Could you check a few things on this model? Use its own coordinates, in mm. A direction names the side the tool comes from. Give positions to 0.01 mm unless a question says otherwise; leave off trailing zeros. Write each loop counter-clockwise with the first axis right and the second up, starting at its lowest first coordinate (ties: lowest second). Pieces come first, ordered by that corner, then holes. Notation, with made-up numbers: M 18,38 L 48,38 A36 ccw 48,75 Z; hole C 40.5,-12.75 d5. An arc over 180 degrees is marked long. One line per item, written item: value.
```python
from build123d import *

# Parameters (mm, degrees)
ESQUISSE1_W             = 52
ESQUISSE1_H             = 44.3
BOSS_EXTRU_1_DEPTH      = 22.3
ESQUISSE4_W             = 38.9
ESQUISSE4_H             = 16.9
ENL_V_MAT_EXTRU_2_DEPTH = 52
BOSS_EXTRU_3_DEPTH      = 44.3
ESQUISSE9_W             = 5.32335475
ESQUISSE9_H             = 32.7
BOSS_EXTRU_4_DEPTH      = 4
ESQUISSE10_W            = 32.7
ESQUISSE10_H            = 4
BOSS_EXTRU_5_DEPTH      = 14.5
ESQUISSE11_W            = 6.122616958
ESQUISSE11_H            = 32.7
BOSS_EXTRU_6_DEPTH      = 4
ESQUISSE12_W            = 32.660291113
ESQUISSE12_H            = 4
BOSS_EXTRU_7_DEPTH      = 14.5
CONG_1_R                = 10
CONG_2_R                = 10
CONG_3_R                = 10
CONG_4_R                = 10


with BuildPart() as part:
    # Esquisse1 → Boss.-Extru.1 (new body)
    with BuildSketch(Plane(origin=(0, 0, 0), x_dir=(1, 0, 0), z_dir=(0, 1, 0))):
        with Locations((-7.759163987, 0)):
            Rectangle(ESQUISSE1_W, ESQUISSE1_H)
    extrude(amount=BOSS_EXTRU_1_DEPTH)

    # Esquisse4 → Enlèv. mat.-Extru.2 (cut)
    with BuildSketch(Plane(origin=(18.240836013, 0, 0), x_dir=(0, 0, -1), z_dir=(1, 0, 0))):
        with Locations((0, 11.15)):
            Rectangle(ESQUISSE4_W, ESQUISSE4_H)
    extrude(amount=-ENL_V_MAT_EXTRU_2_DEPTH, mode=Mode.SUBTRACT)

    # Esquisse5 → Boss.-Extru.3 (add)
    with BuildSketch(Plane.XY.offset(22.15)):
        with BuildLine():
            Line((-33.759163987, 22.3), (-33.759163987, 0))
            ThreePointArc((-33.759163987, 0), (-44.909163987, 11.15), (-33.759163987, 22.3))
        make_face()
    extrude(amount=-BOSS_EXTRU_3_DEPTH)

    # Esquisse9 → Boss.-Extru.4 (add)
    with BuildSketch(Plane.XZ):
        with Locations((15.579158638, 0)):
            Rectangle(ESQUISSE9_W, ESQUISSE9_H)
    extrude(amount=BOSS_EXTRU_4_DEPTH)

    # Esquisse10 → Boss.-Extru.5 (add)
    with BuildSketch(Plane(origin=(18.240836013, 0, 0), x_dir=(0, 0, -1), z_dir=(1, 0, 0))):
        with Locations((0, -2)):
            Rectangle(ESQUISSE10_W, ESQUISSE10_H)
    extrude(amount=BOSS_EXTRU_5_DEPTH)

    # Esquisse11 → Boss.-Extru.6 (add)
    with BuildSketch(Plane(origin=(0, 22.3, 0), x_dir=(1, 0, 0), z_dir=(0, 1, 0))):
        with Locations((15.179527534, 0)):
            Rectangle(ESQUISSE11_W, ESQUISSE11_H)
    extrude(amount=BOSS_EXTRU_6_DEPTH)

    # Esquisse12 → Boss.-Extru.7 (add)
    with BuildSketch(Plane(origin=(18.240836013, 0, 0), x_dir=(0, 0, -1), z_dir=(1, 0, 0))):
        with Locations((0.019854443, 24.3)):
            Rectangle(ESQUISSE12_W, ESQUISSE12_H)
    extrude(amount=BOSS_EXTRU_7_DEPTH)

    # Congé1
    # the kernel refuses this fillet: 10 mm, written as the material it takes off along each edge
    with BuildSketch(Plane(origin=(12.917481263, -4, -36.35), x_dir=(1, 0, 0), z_dir=(0, 0, 1))) as cong_1_piece_1:
        with BuildLine():
            CenterArc((8, 10), CONG_1_R, 216.869897646, 53.130102354)
            Line((0, 4), (-0.16, 3.88))
            ThreePointArc((-0.16, 3.88), (-0.2, 2), (-0.2, 0))
            Line((-0.2, 0), (0, -0.2))
            Line((0, -0.2), (8, -0.2))
            Line((8, -0.2), (8, 0))
        make_face()
    extrude(amount=72.7, mode=Mode.SUBTRACT)

    # Congé2
    # the kernel refuses this fillet: 10 mm, written as the material it takes off along each edge
    with BuildSketch(Plane(origin=(12.118219055, 26.3, 36.35), x_dir=(1, 0, 0), z_dir=(0, 0, -1))) as cong_2_piece_1:
        with BuildLine():
            CenterArc((8, 10), CONG_2_R, 216.869897646, 53.130102354)
            Line((0, 4), (-0.16, 3.88))
            ThreePointArc((-0.16, 3.88), (-0.2, 2), (-0.2, 0))
            Line((-0.2, 0), (0, -0.2))
            Line((0, -0.2), (8, -0.2))
            Line((8, -0.2), (8, 0))
        make_face()
    extrude(amount=72.7, mode=Mode.SUBTRACT)

    # Congé3
    # the kernel refuses this fillet: 10 mm, written as the material it takes off along each edge
    with BuildSketch(Plane(origin=(32.740836013, -4, -36.35), x_dir=(-1, 0, 0), z_dir=(0, 0, 1))) as cong_3_piece_1:
        with BuildLine():
            CenterArc((8, -10), CONG_3_R, 90, 53.130102354)
            Line((0, -4), (-0.16, -3.88))
            ThreePointArc((-0.16, -3.88), (-0.2, -2), (-0.2, 0))
            Line((-0.2, 0), (0, 0.2))
            Line((0, 0.2), (8, 0.2))
            Line((8, 0.2), (8, 0))
        make_face()
    extrude(amount=72.7, mode=Mode.SUBTRACT)

    # Congé4
    # the kernel refuses this fillet: 10 mm, written as the material it takes off along each edge
    with BuildSketch(Plane(origin=(32.740836013, 26.3, -36.35), x_dir=(0, -1, 0), z_dir=(0, 0, 1))) as cong_4_piece_1:
        with BuildLine():
            CenterArc((10, -8), CONG_4_R, 126.869897646, 53.130102354)
            Line((0, -8), (-0.2, -8))
            Line((-0.2, -8), (-0.2, 0))
            Line((-0.2, 0), (0, 0.2))
            ThreePointArc((0, 0.2), (2, 0.2), (3.88, 0.16))
            Line((3.88, 0.16), (4, 0))
        make_face()
    extrude(amount=72.660291113, mode=Mode.SUBTRACT)


solid = part.part
```
1) We'd pull the mould along Z, two halves only. Please class faces 6 (the face through (23, -2, 16.35)), 7 (the face through (23, -4, 0)), 8 (the face through (-7, 2.7, 0)): pulls with the +Z half, pulls with the -Z half, needs draft (parallel to the pull), parting line crosses it, or undercut.
Outcome:
face 6: pulls with the +Z half
face 7: needs draft
face 8: undercut
2) On a 3-axis mill with a long thin cutter (end or side, diameter ignored), from which of +Z, -Z, +X, -X, +Y, -Y can I reach the whole of each face in a straight line? I mean faces 1 (the face through (23, -2, -16.35)), 2 (the face through (16.387, -2.915, -0.229)), 3 (the face through (22, 24, -16.35)), 4 (the face through (-33.759, 11, 0)), 5 (the face through (25, 22.3, 0)). Say none if no direction works.
Outcome:
face 1: -Z, +X, -X, -Y
face 2: +Z, -Z, -X, -Y
face 3: -Z, +X, -X, +Y
face 4: +X
face 5: +Z, -Z, +X
3) If we section it at C-C, the plane z = -15.5: Write out the boundary of the cut face in (x, y).
Outcome:
outline: M -33.76,0 L 12.92,0 A10 ccw 20.92,-4 L 24.74,-4 A10 ccw 32.74,0 L 18.24,0 L 18.24,2.7 L -33.76,2.7 L -33.76,19.6 L 18.24,19.6 L 18.24,22.3 L 32.74,22.3 A10 ccw 24.74,26.3 L 20.12,26.3 A10 ccw 12.12,22.3 L -33.76,22.3 A11.15 ccw Z
4) If we section it at D-D, the plane y = 11.15: Write out the boundary of the cut face in (x, z), then the cut area to 3 significant figures.
Outcome:
outline: M -44.91,-22.15 L 18.24,-22.15 L 18.24,-19.45 L -33.76,-19.45 L -33.76,19.45 L 18.24,19.45 L 18.24,22.15 L -44.91,22.15 Z
area: 775 mm^2
5) If we section it at A-A, the plane x = 23.5: Write out the boundary of the cut face in (y, z), then the cut area to 3 significant figures.
Outcome:
outline: M -4,-16.35 L 0,-16.35 L 0,16.35 L -4,16.35 Z; M 22.3,-16.35 L 26.3,-16.35 L 26.3,16.31 L 22.3,16.31 Z
area: 261 mm^2
6) If we section it at B-B, the plane x = -2: Write out the boundary of the cut face in (y, z).
Outcome:
outline: M 0,-22.15 L 22.3,-22.15 L 22.3,22.15 L 0,22.15 Z; hole M 2.7,-19.45 L 19.6,-19.45 L 19.6,19.45 L 2.7,19.45 Z
7) Please list where these lines run through material, in increasing order: L1, parallel to Z at x = -21.5, y = 18; L2, parallel to Y at x = 17, z = -17. Write a range as from..to.
Outcome:
L1: z = -22.15..-19.45, 19.45..22.15
L2: y = 0..2.7, 19.6..22.3
8) I'm going to push flat-ended pins straight in: pin 1 (11.5 mm diameter, centred on x = 28, z = 7.5, fed in from +Y); pin 2 (1.5 mm diameter, centred on x = 7, z = -2.5, fed in from -Y); pin 3 (5 mm diameter, centred on y = 13, z = -1.5, fed in from +X); pin 4 (4.5 mm diameter, centred on x = 24.5, y = 25, fed in from +Z). Where does each tip first touch, or does it pass through?
Outcome:
pin 1: stops at y = 26.3
pin 2: stops at y = 0
pin 3: stops at x = -33.76
pin 4: stops at z = 16.31
